Read the model definition and answer for the solid it produces. Units are mm, in the model's axes. Face numbers are marked on the shaded views. A direction names the side the tool comes from. Round coordinates to 2 decimals unless told otherwise and drop trailing zeros. Order: outer loops, then holes, each group sorted by start corner. A loop starts at its lowest first (then second) coordinate and runs counter-clockwise, first axis right, second up.
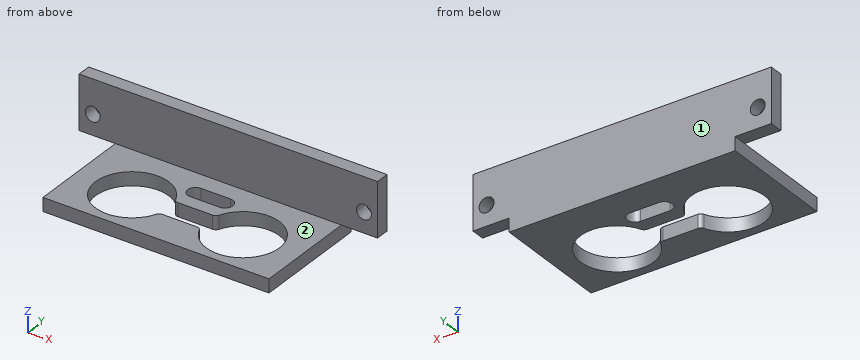
from build123d import *

# Parameters (mm, degrees)
SKETCH_1_W          = 50
SKETCH_1_H          = 20
EXTRUDE_1_DEPTH     = 3
SKETCH_2_W          = 50
SKETCH_2_H          = 15
EXTRUDE_2_DEPTH     = 6
SKETCH_5_W          = 50
SKETCH_5_H          = 12
CUT_EXTRUDE_2_DEPTH = 3
SKETCH_6_W          = 8
SKETCH_6_H          = 12
SKETCH_6_R          = 1.65
EXTRUDE_3_DEPTH     = 3


with BuildPart() as part:
    # 草图1 → 凸台-拉伸1 (new body)
    with BuildSketch(Plane.XY):
        Rectangle(SKETCH_1_W, SKETCH_1_H)
        with BuildLine():
            Line((-3.85, 2.5), (3.85, 2.5))
            ThreePointArc((3.85, 2.5), (4.404700196, 2.667949706), (4.773076923, 3.115384615))
            ThreePointArc((4.773076923, 3.115384615), (20.35, 0), (4.773076923, -3.115384615))
            ThreePointArc((4.773076923, -3.115384615), (4.404700196, -2.667949706), (3.85, -2.5))
            Line((3.85, -2.5), (-3.85, -2.5))
            ThreePointArc((-3.85, -2.5), (-4.404700196, -2.667949706), (-4.773076923, -3.115384615))
            ThreePointArc((-4.773076923, -3.115384615), (-20.35, 0), (-4.773076923, 3.115384615))
            ThreePointArc((-4.773076923, 3.115384615), (-4.404700196, 2.667949706), (-3.85, 2.5))
        make_face(mode=Mode.SUBTRACT)
        with BuildLine():
            Line((3.25, 5.5), (-3.25, 5.5))
            ThreePointArc((-3.25, 5.5), (-5, 7.25), (-3.25, 9))
            Line((-3.25, 9), (3.25, 9))
            ThreePointArc((3.25, 9), (5, 7.25), (3.25, 5.5))
        make_face(mode=Mode.SUBTRACT)
    extrude(amount=EXTRUDE_1_DEPTH)

    # 草图2 → 凸台-拉伸2 (add)
    with BuildSketch(Plane(origin=(0, 10, 0), x_dir=(1, 0, 0), z_dir=(0, 1, 0))):
        with Locations((0, -7.5)):
            Rectangle(SKETCH_2_W, SKETCH_2_H)
    extrude(amount=EXTRUDE_2_DEPTH)

    # 草图5 → 切除-拉伸2 (cut)
    with BuildSketch(Plane.XZ.offset(-10)):
        with Locations((0, 9)):
            Rectangle(SKETCH_5_W, SKETCH_5_H)
    extrude(amount=-CUT_EXTRUDE_2_DEPTH, mode=Mode.SUBTRACT)

    # 草图6 → 凸台-拉伸3 (add)
    with BuildSketch(Plane(origin=(0, 16, 0), x_dir=(1, 0, 0), z_dir=(0, 1, 0))):
        with Locations((29, -9)):
            Rectangle(SKETCH_6_W, SKETCH_6_H)
        with Locations((30, -7.5)):
            Circle(SKETCH_6_R, mode=Mode.SUBTRACT)
        with Locations((-29, -9)):
            Rectangle(SKETCH_6_W, SKETCH_6_H)
        with Locations((-30, -7.5)):
            Circle(SKETCH_6_R, mode=Mode.SUBTRACT)
    extrude(amount=-EXTRUDE_3_DEPTH)


solid = part.part
Q1. A cutting plane is placed at B-B, the plane x = -12.25. Give the vertices of the cut face in (y, z), plus the area to 3 significant figures.
Outcome:
outline: (-10, 0) - (-8.1, 0) - (-8.1, 3) - (-10, 3) - close; (8.1, 0) - (16, 0) - (16, 15) - (13, 15) - (13, 3) - (8.1, 3) - close
area: 65.4 mm2
Q2. Flat-ended cylindrical pins translate along their axes: pin 1 (8 mm diameter, centred on x = -0.5, y = 2.5, fed in from +Z); pin 2 (3.5 mm diameter, centred on y = 4, z = 2, fed in from -X); pin 3 (2.5 mm diameter, centred on x = 30.5, y = 15, fed in from -Z). Find the tip coordinate at first contact, or state that the pin passes through.
Outcome:
pin 1: stops at z = 3
pin 2: stops at x = -25
pin 3: stops at z = 3
Q3. For the marked faces 1 and 2, determine the directions among +Z, -Z, +X, -X, +Y, -Y from which every point of the face is accessible in a straight line to the end or side of a thin tool.
Outcome:
face 1: +Z, -Z, +X, -X, +Y
face 2: +Z, +X, -X, -Y
Q4. Straight lines are drawn through the part: probe 1 along X at (y, z) = (15.1, 7.5); probe 2 along Z at (x, y) = (-30, 15.15); probe 3 along Y at (x, z) = (12.25, 1.8). For each, find the intervals that lie inside material, in ascending order.
Outcome:
probe 1: x = -33 to -31.65, -28.35 to 28.35, 31.65 to 33
probe 2: z = 3 to 5.85, 9.15 to 15
probe 3: y = -10 to -8.1, 8.1 to 16
Q5. A cutting plane is placed at D-D, the plane z = 1.75. Give the vertices of the cut face in (x, y), plus the area to 3 significant figures.
Outcome:
outline: (-25, -10) - (25, -10) - (25, 16) - (-25, 16) - close; hole (-4.77, -3.12) arc R1 cw to (-3.85, -2.5) - (3.85, -2.5) arc R1 cw to (4.77, -3.12) arc R8.1 ccw (long way) to (4.77, 3.12) arc R1 cw to (3.85, 2.5) - (-3.85, 2.5) arc R1 cw to (-4.77, 3.12) arc R8.1 ccw (long way) to start; hole (-3.25, 5.5) - (3.25, 5.5) arc R1.75 ccw to (3.25, 9) - (-3.25, 9) arc R1.75 ccw to start
area: 812 mm2
Q6. A cutting plane is placed at A-A, the plane z = 7.5. Give the vertices of the cut face in (x, y), plus the area to 3 significant figures.
Outcome:
outline: (-33, 13) - (-31.65, 13) - (-31.65, 16) - (-33, 16) - close; (-28.35, 13) - (28.35, 13) - (28.35, 16) - (-28.35, 16) - close; (31.65, 13) - (33, 13) - (33, 16) - (31.65, 16) - close
area: 178 mm2
Q7. A cutting plane is placed at C-C, the plane y = 0. Give the vertices of the cut face in (x, z).
Outcome:
outline: (-25, 0) - (-20.35, 0) - (-20.35, 3) - (-25, 3) - close; (20.35, 0) - (25, 0) - (25, 3) - (20.35, 3) - close
